Geometry check sheet. Reference: drawing and pictorial views, mm from the part's lowest x, y, z. A direction names the side the tool comes from. Give positions to 0.01 mm unless a question says otherwise; leave off trailing zeros. Order: outer loops, then holes, each group sorted by start corner. A loop starts at its lowest first (then second) coordinate and runs counter-clockwise, first axis right, second up.
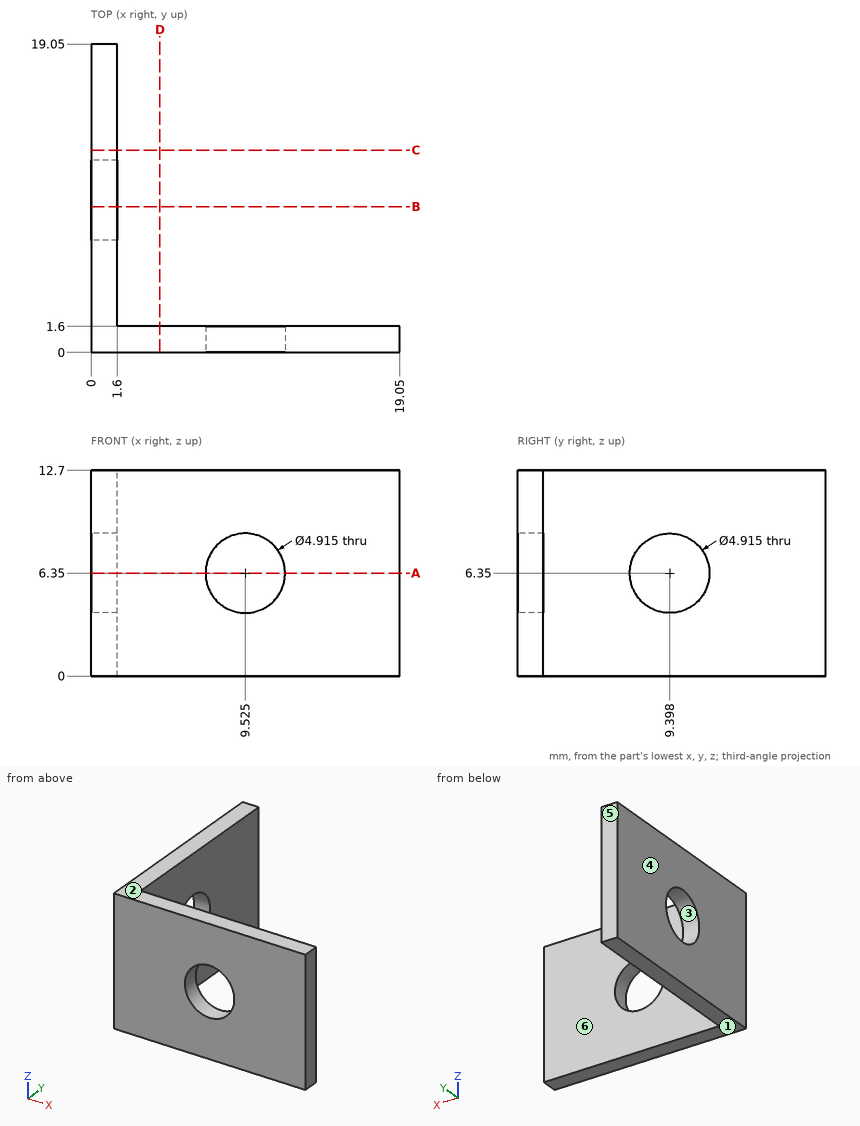
1) Section check A-A, the plane z = 6.35. Record the cut outline in (x, y), then the cut area to 3 significant figures.
Recorded:
outline: (0, 0) - (7.07, 0) - (7.07, 1.6) - (1.6, 1.6) - (1.6, 6.94) - (0, 6.94) - close; (0, 11.86) - (1.6, 11.86) - (1.6, 19.05) - (0, 19.05) - close; (11.98, 0) - (19.05, 0) - (19.05, 1.6) - (11.98, 1.6) - close
area: 42.7 mm2
2) Draft check along Z on the marked faces 1, 2, 3 and 4. Enter one of: +Z half, -Z half, draft (parallel to the pull), parting line (faces both ways), or undercut.
Recorded:
face 1: -Z half
face 2: +Z half
face 3: undercut
face 4: draft
3) Set-up check for the marked faces 5 and 6: record each of +Z, -Z, +X, -X, +Y, -Y from which the full face is reachable in a straight line by a thin tool's end or side.
Recorded:
face 5: +Z, -Z, +X, -X, +Y
face 6: +Z, -Z, +X, +Y
4) Material ranges on L1, parallel to X at y = 8.5, z = 10.5; L2, parallel to Y at x = 1.3, z = 6.35, recorded low to high.
Recorded:
L1: x = 0 to 1.6
L2: y = 0 to 6.94, 11.86 to 19.05
5) Depth check by flat-ended pin: pin 1 Ø3 at (y, z) = (10, 5) entering from +X; pin 2 Ø6.5 at (x, z) = (7, 5) entering from +Y. Enter the tip coordinate at first touch or a pass-through.
Recorded:
pin 1: stops at x = 1.6
pin 2: stops at y = 1.6
6) Section check C-C, the plane y = 12.5. Record the cut outline in (x, z), then the cut area to 3 significant figures.
Recorded:
outline: (0, 0) - (1.6, 0) - (1.6, 12.7) - (0, 12.7) - close
area: 20.3 mm2
7) Section check B-B, the plane y = 9. Record the cut outline in (x, z) (1 decimal).
Recorded:
outline: (0, 0) - (1.6, 0) - (1.6, 3.9) - (0, 3.9) - close; (0, 8.8) - (1.6, 8.8) - (1.6, 12.7) - (0, 12.7) - close
